Part model, mm, in its own coordinate system. A direction names the side the tool comes from. Give positions to 0.01 mm unless a question says otherwise; leave off trailing zeros. Write item = value, one per line. Start each with the question number.
Item 1: Flat gauge pins, fed straight in: P1, Ø4, axis at x = 22.1, z = 22.1, coming from the +Y side; P2, Ø1.5, axis at y = 7, z = -23.5, coming from the -X side; P3, Ø1.8, axis at y = 9.5, z = -2, coming from the -X side. Where does each tip first touch, or does it go through?
Item 2: Drill centre lines: line 1 along X through (y, z) = (2.5, 19); line 2 along X through (y, z) = (9.75, 21); line 3 along X through (y, z) = (10.5, -22.5). Where is each one in solid material? Low to high.
Item 3: Band-saw the part on A-A on y = 12. Count the separate pieces of the cut face and the enclosed holes in it, plus the area to 3 significant figures.
Item 4: Tool access for faces 1 (the face through (-3.62, 7.96, -6.16)), 2 (the face through (1, 4.6, -33)), 3 (the face through (-20.84, 3.79, 20.95)): list every direction of +Z, -Z, +X, -X, +Y, -Y with a clear straight run to the whole face (end or side of a thin tool).
```python
from build123d import *

# Parameters (mm, degrees)
SKETCH1_R               = 37
SKETCH1_R_2             = 1
BOSS_EXTRUDE1_DEPTH     = 14
F_3_8_CLEARANCE_HOLE1_D = 10.31748
SKETCH8_R               = 34.1
SKETCH8_R_2             = 28.4
CUT_EXTRUDE3_DEPTH      = 3
SKETCH9_R               = 22.5
CUT_EXTRUDE4_DEPTH      = 5
CUT_EXTRUDE2_DEPTH      = 6
CHAMFER1_SIZE           = 0.8
CIRPATTERN1_COUNT       = 8


with BuildPart() as part:
    # Sketch1 → Boss-Extrude1 (new body)
    with BuildSketch(Plane(origin=(0, 0, 0), x_dir=(1, 0, 0), z_dir=(0, 1, 0))):
        with Locations(Location((0, 0, 0), (0, 0, 270))):
            Circle(SKETCH1_R)
        with Locations(Location((0, 31.25, 0), (0, 0, 270))):
            Circle(SKETCH1_R_2, mode=Mode.SUBTRACT)
        with Locations(Location((22.097086912, 22.097086912, 0), (0, 0, 270))):
            Circle(SKETCH1_R_2, mode=Mode.SUBTRACT)
        with Locations(Location((31.25, 0, 0), (0, 0, 270))):
            Circle(SKETCH1_R_2, mode=Mode.SUBTRACT)
        with Locations(Location((22.097086912, -22.097086912, 0), (0, 0, 270))):
            Circle(SKETCH1_R_2, mode=Mode.SUBTRACT)
        with Locations(Location((0, -31.25, 0), (0, 0, 270))):
            Circle(SKETCH1_R_2, mode=Mode.SUBTRACT)
        with Locations(Location((-22.097086912, -22.097086912, 0), (0, 0, 270))):
            Circle(SKETCH1_R_2, mode=Mode.SUBTRACT)
        with Locations(Location((-31.25, 0, 0), (0, 0, 270))):
            Circle(SKETCH1_R_2, mode=Mode.SUBTRACT)
        with Locations(Location((-22.097086912, 22.097086912, 0), (0, 0, 270))):
            Circle(SKETCH1_R_2, mode=Mode.SUBTRACT)
    extrude(amount=BOSS_EXTRUDE1_DEPTH)

    # 3/8 Clearance Hole1 (through all)
    with Locations(Plane(origin=(0, 0, 0), x_dir=(-1, 0, 0), z_dir=(0, -1, 0))):
        with Locations((0, 0)):
            Hole(F_3_8_CLEARANCE_HOLE1_D / 2)

    # Sketch8 → Cut-Extrude3 (cut)
    with BuildSketch(Plane.XZ):
        with Locations(Location((0, 0, 0), (0, 0, 270))):
            Circle(SKETCH8_R)
        with Locations(Location((0, 0, 0), (0, 0, 270))):
            Circle(SKETCH8_R_2, mode=Mode.SUBTRACT)
    extrude(amount=-CUT_EXTRUDE3_DEPTH, mode=Mode.SUBTRACT)

    # Sketch9 → Cut-Extrude4 (cut)
    with BuildSketch(Plane.XZ):
        with Locations(Location((0, 0, 0), (0, 0, 270))):
            Circle(SKETCH9_R)
    extrude(amount=-CUT_EXTRUDE4_DEPTH, mode=Mode.SUBTRACT)

    # Sketch7 → Cut-Extrude2 (cut)
    with BuildSketch(Plane.XZ.offset(-5)):
        Polygon((0, 8.248891971), (-7.14375, 4.124445986), (-7.14375, -4.124445986), (0, -8.248891971), (7.14375, -4.124445986), (7.14375, 4.124445986), align=None)
    extrude(amount=-CUT_EXTRUDE2_DEPTH, mode=Mode.SUBTRACT)

    # Chamfer1
    chamfer1_edges = [part.edges().sort_by_distance(p)[0] for p in [
        (0, 0, 34.1),
        (0, 0, 28.4),
    ]]
    chamfer(chamfer1_edges, length=CHAMFER1_SIZE)

    # Sketch10 → Cut-Revolve1 (revolve, cut)
    with BuildSketch(Plane(origin=(0, 0, 0), x_dir=(0, 0, -1), z_dir=(1, 0, 0))):
        Polygon((32.95, 4.6), (32.95, 3), (31.25, 3), (31.25, 14), (33.85, 14), (33.85, 4.6), align=None)
    cut_revolve1 = revolve(axis=Axis((0, 14, -31.25), (0, 1, 0)), mode=Mode.SUBTRACT)

    # CirPattern1: Cut-Revolve1 ×8 about axis
    cirpattern1_axis = Axis((0, 0, 0), (0, 1, 0))
    for i in range(1, CIRPATTERN1_COUNT):
        add(cut_revolve1.rotate(cirpattern1_axis, i * 360 / CIRPATTERN1_COUNT), mode=Mode.SUBTRACT)


solid = part.part
```
Values found:
q1.P1 = 4.6
q1.P2 = -29.18
q1.P3 = -36.98
q2.line_1 = -31.75 to -28.32, -21.11 to -12.05, 12.05 to 21.11, 28.32 to 31.75
q2.line_2 = -30.46 to -24.45, -19.74 to 19.74, 24.45 to 30.46
q2.line_3 = -29.37 to -24.67, -19.53 to 19.53, 24.67 to 29.37
q3.separate_pieces = 1
q3.enclosed_holes = 9
q3.area = 4,050 mm^2
q4.face_1 = -Y
q4.face_2 = +Y
q4.face_3 = +Y, -Y
